Geometry: final body of the model. Coordinates: model frame, mm. Face numbers are marked on the shaded views. Give positions to 0.01 mm unless a question says otherwise; leave off trailing zeros. Write each loop counter-clockwise with the first axis right and the second up, starting at its lowest first coordinate (ties: lowest second). Pieces come first, ordered by that corner, then holes. Notation, with made-up numbers: M 50.5,15 L 78.5,15 A20 ccw 78.5,38 Z; hole C 50.25,-39.75 d10. An arc over 180 degrees is marked long. Use one line per item in the form item = value. Start each with the question number.
Item 1: Section query A-A on x = -65. Return loops of the section in (y, z).
Item 2: Contact query for flat-ended pins moving along their axis: P1, Ø12, axis at x = -121, y = 17.5, coming from the -Z side; P2, Ø5, axis at x = -51, y = 11, coming from the +Z side; P3, Ø8, axis at y = 21.5, z = -3.5, coming from the -X side; P4, Ø8, axis at x = -132, y = 3, coming from the +Z side. Output: stop coordinate, or through.
Item 3: Pull-direction query (Z, two-part tool) for the marked faces 1, 2 and 3; classes: released by +Z, released by -Z, zero draft, split by the parting line, or undercut.
Item 4: Section query D-D on y = 15. Return loops of the section in (x, z).
Item 5: Section query C-C on z = -25. Return loops of the section in (x, y).
Item 6: Section query B-B on y = 7.5. Return loops of the section in (x, z), then the cut area to 3 significant figures.
Item 7: Material intervals for line 1 along Z through (x, y) = (-28, 19); line 2 along X through (y, z) = (-2, -39.5); line 3 along Y through (x, z) = (-136.5, -4), sorted ascending. Write a range as from..to.
from build123d import *

# Parameters (mm, degrees)
BOSS_EXTRUDE1_DEPTH        = 5
BOSS_EXTRUDE1_DEPTH_BACK   = 46
SKETCH1_R                  = 2.5
BOSS_EXTRUDE1_2_DEPTH      = 5
BOSS_EXTRUDE1_2_DEPTH_BACK = 46
BOSS_EXTRUDE1_3_DEPTH      = 5
BOSS_EXTRUDE1_3_DEPTH_BACK = 46
BOSS_EXTRUDE1_4_DEPTH      = 5
BOSS_EXTRUDE1_4_DEPTH_BACK = 46
BOSS_EXTRUDE1_5_DEPTH      = 5
BOSS_EXTRUDE1_5_DEPTH_BACK = 46
BOSS_EXTRUDE2_DEPTH        = 41


with BuildPart() as part:
    # Sketch1 → Boss-Extrude1 (new, two sides: drawn at the far end of the back side and taken through both)
    with BuildSketch(Plane.XY.offset(-BOSS_EXTRUDE1_DEPTH_BACK)):
        Circle(SKETCH1_R)
    extrude(amount=BOSS_EXTRUDE1_DEPTH + BOSS_EXTRUDE1_DEPTH_BACK)



with BuildPart() as body_2:
    # Sketch1 → Boss-Extrude1 2 (new, two sides: drawn at the far end of the back side and taken through both)
    with BuildSketch(Plane.XY.offset(-BOSS_EXTRUDE1_2_DEPTH_BACK)):
        with Locations((0, 15)):
            Circle(SKETCH1_R)
    extrude(amount=BOSS_EXTRUDE1_2_DEPTH + BOSS_EXTRUDE1_2_DEPTH_BACK)


with BuildPart() as body_3:
    # Sketch1 → Boss-Extrude1 3 (new, two sides: drawn at the far end of the back side and taken through both)
    with BuildSketch(Plane.XY.offset(-BOSS_EXTRUDE1_3_DEPTH_BACK)):
        with Locations((-130, 15)):
            Circle(SKETCH1_R)
    extrude(amount=BOSS_EXTRUDE1_3_DEPTH + BOSS_EXTRUDE1_3_DEPTH_BACK)


with BuildPart() as body_4:
    # Sketch1 → Boss-Extrude1 4 (new, two sides: drawn at the far end of the back side and taken through both)
    with BuildSketch(Plane.XY.offset(-BOSS_EXTRUDE1_4_DEPTH_BACK)):
        with Locations((-130, 0)):
            Circle(SKETCH1_R)
    extrude(amount=BOSS_EXTRUDE1_4_DEPTH + BOSS_EXTRUDE1_4_DEPTH_BACK)


with BuildPart() as body_5:
    # Sketch1 → Boss-Extrude1 5 (new, two sides: drawn at the far end of the back side and taken through both)
    with BuildSketch(Plane.XY.offset(-BOSS_EXTRUDE1_5_DEPTH_BACK)):
        with Locations((-65, 7.5)):
            Circle(SKETCH1_R)
    extrude(amount=BOSS_EXTRUDE1_5_DEPTH + BOSS_EXTRUDE1_5_DEPTH_BACK)


with BuildPart() as part_1:
    add(part.part)

    add(body_2.part)  # Boss-Extrude2 merges body 2

    add(body_3.part)  # Boss-Extrude2 merges body 3

    add(body_4.part)  # Boss-Extrude2 merges body 4

    add(body_5.part)  # Boss-Extrude2 merges body 5
    # Sketch2 → Boss-Extrude2 (add)
    with BuildSketch(Plane.XY):
        with BuildLine():
            Line((-130, 27.5), (0, 27.5))
            ThreePointArc((0, 27.5), (20, 7.5), (0, -12.5))
            Line((0, -12.5), (-130, -12.5))
            ThreePointArc((-130, -12.5), (-150, 7.5), (-130, 27.5))
        make_face()
    extrude(amount=-BOSS_EXTRUDE2_DEPTH)


solid = part_1.part
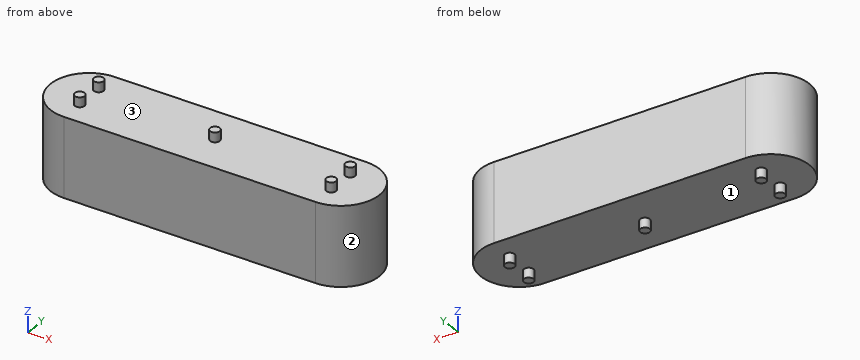
Answer sheet:
q1.outline = M -12.5,-41 L 5,-41 L 5,-46 L 10,-46 L 10,-41 L 27.5,-41 L 27.5,0 L 10,0 L 10,5 L 5,5 L 5,0 L -12.5,0 Z
q2.P1 = -41
q2.P2 = 0
q2.P3 = -147.32
q2.P4 = 5
q3.face_1 = released by -Z
q3.face_2 = zero draft
q3.face_3 = released by +Z
q4.outline = M -148.54,-41 L -132.5,-41 L -132.5,-46 L -127.5,-46 L -127.5,-41 L -2.5,-41 L -2.5,-46 L 2.5,-46 L 2.5,-41 L 18.54,-41 L 18.54,0 L 2.5,0 L 2.5,5 L -2.5,5 L -2.5,0 L -127.5,0 L -127.5,5 L -132.5,5 L -132.5,0 L -148.54,0 Z
q5.outline = M -130,-12.5 L 0,-12.5 A20 ccw 0,27.5 L -130,27.5 A20 ccw Z
q6.outline = M -150,-41 L -67.5,-41 L -67.5,-46 L -62.5,-46 L -62.5,-41 L 20,-41 L 20,0 L -62.5,0 L -62.5,5 L -67.5,5 L -67.5,0 L -150,0 Z
q6.area = 7,020 mm2
q7.line_1 = -41..0
q7.line_2 = -147.6..17.6
q7.line_3 = -11.41..26.41
